The model under review builds one solid part; all positions refer to its coordinate system, in mm. A direction names the side the tool comes from. Round coordinates to 2 decimals unless told otherwise and drop trailing zeros. Write each loop counter-clockwise with the first axis right and the second up, starting at its lowest first coordinate (ties: lowest second). Pieces come first, ordered by that corner, then holes. Notation, with made-up numbers: M 50.25,85.5 L 66.25,85.5 A14 ccw 66.25,91.5 Z; hole C 50.5,30 d5. An arc over 180 degrees is marked long. Write item = value, one per line. Start each with the question number.
Item 1: Tool access review of faces 1 (the flat face through (5, 9.654, 32)), 2 (the flat face through (6, 12.888, 19)): name each direction out of +Z, -Z, +X, -X, +Y, -Y from which nothing blocks a thin tool from reaching the whole face with its end or side.
Item 2: Take a section at B-B, the plane y = -3.75. Give the boundary of the cut face in (x, z), plus the area to 3 significant figures.
Item 3: For pin 1 Ø4 at (x, y) = (5, 4) entering from +Z, flat-tipped, find the tip position at first contact; note if it passes through.
Item 4: To check wall thickness, follow line 1 along X through (y, z) = (7.25, 31.5); line 2 along Y through (x, z) = (-4.5, 34.5); line 3 along Z through (x, y) = (-11.5, -6.25). State the ranges of each line that lie inside material, in increasing order.
Item 5: Take a section at C-C, the plane x = -5. Give the boundary of the cut face in (y, z), plus the area to 3 significant figures.
Item 6: The part is to be moulded in two halves that separate along X. For faces 3 (the flat face through (31.454, 0, 19)), 4 (the flat face through (5, 0, 25.4)), 5 (the flat face through (26.997, 0, 32)), 6 (the flat face through (-19.346, 0, 19)), say which applies: +X half, -X half, draft (parallel to the pull), parting line (faces both ways), or undercut.
Item 7: Take a section at A-A, the plane z = 29. Give the boundary of the cut face in (x, y).
from build123d import *

# Parameters (mm, degrees)
F0_W     = 50.8
F0_H     = 25.4
F1_DEPTH = 25.4
F2_W     = 3.4749715865
F2_H     = 3.2341817119
F2_W_2   = 42.8683459759
F2_H_2   = 19.3071160465
F2_W_3   = 4.4566824377
F2_H_3   = 2.8587022416
F3_DEPTH = 12.7


with BuildPart() as f1:
    # F0 (on Top) → F1 (new body)
    with BuildSketch(Plane.XY):
        with Locations((6.0539245605, 0.1877397351)):
            Rectangle(F0_W, F0_H)
    extrude(amount=F1_DEPTH)

    # F2 (on face) → F3 (join)
    with BuildSketch(Plane.XY.offset(25.4)):
        with Locations((-17.6085896462, 11.2706488792)):
            Rectangle(F2_W, F2_H)
        with Locations((5.563069135, 11.2706488792)):
            Rectangle(F2_W_2, F2_H)
        with Locations((-17.6085896462, 0)):
            Rectangle(F2_W, F2_H_2)
        with Locations((29.2255833417, 11.2706488792)):
            Rectangle(F2_W_3, F2_H)
        with Locations((-17.6085896462, -11.0829091441)):
            Rectangle(F2_W, F2_H_3)
        with Locations((29.2255833417, 0)):
            Rectangle(F2_W_3, F2_H_2)
        with Locations((5.563069135, -11.0829091441)):
            Rectangle(F2_W_2, F2_H_3)
        with Locations((29.2255833417, -11.0829091441)):
            Rectangle(F2_W_3, F2_H_3)
    extrude(amount=F3_DEPTH)


solid = f1.part
Response values:
q1.face_1 = +Z
q1.face_2 = +Z, -Z, +X, -X, +Y
q2.outline = M -19.35,0 L 31.45,0 L 31.45,38.1 L 27,38.1 L 27,25.4 L -15.87,25.4 L -15.87,38.1 L -19.35,38.1 Z
q2.area = 1,390 mm2
q3.pin_1 = 25.4
q4.line_1 = -19.35 to -15.87, 27 to 31.45
q4.line_2 = -12.51 to -9.65, 9.65 to 12.89
q4.line_3 = 0 to 25.4
q5.outline = M -12.51,0 L 12.89,0 L 12.89,38.1 L 9.65,38.1 L 9.65,25.4 L -9.65,25.4 L -9.65,38.1 L -12.51,38.1 Z
q5.area = 723 mm2
q6.face_3 = +X half
q6.face_4 = undercut
q6.face_5 = undercut
q6.face_6 = -X half
q7.outline = M -19.35,-12.51 L 31.45,-12.51 L 31.45,12.89 L -19.35,12.89 Z; hole M -15.87,-9.65 L 27,-9.65 L 27,9.65 L -15.87,9.65 Z
